The figure shows three views and two pictorial views of one solid part (mm, origin at its lowest corner). Answer the questions. Round coordinates to 2 decimals unless told otherwise and drop trailing zeros. Order: outer loops, then holes, each group sorted by start corner. A loop starts at its lowest first (then second) coordinate and runs counter-clockwise, first axis right, second up. Notation, with made-up numbers: (-27.5, -7.5) - (16.5, -7.5) arc R32 ccw to (16.5, 18.5) - close; hole circle Ø6 at (2.5, 30). An arc over 180 degrees is marked (long way). Answer as a JSON object with one key per item and string values. Group by question number.
Q1. Given pin 1 Ø4 at (x, z) = (152.5, 100) entering from -Y; pin 2 Ø2 at (x, y) = (167, 6) entering from -Z (1 decimal); pin 3 Ø6 at (x, y) = (135.5, 4) entering from +Z; pin 4 Ø2 at (y, z) = (7.5, 119) entering from -X, each flat-ended and moving along its own axis, determine where each tip first touches the part or whether it passes through.
Q2. Consider line 1 (X direction, y = 7.5, z = 170); line 2 (X direction, y = 6.25, z = 100) (1 decimal); line 3 (Z direction, x = 152.5, y = 4.5). Determine where each line is inside the solid, lowest interval first.
Q3. A cutting plane is placed at B-B on z = 188. Determine the outline of the cut face in (x, y).
Q4. A cutting plane is placed at C-C on y = 4.25. Determine the outline of the cut face in (x, z).
Q5. A cutting plane is placed at D-D on z = 231. Determine the outline of the cut face in (x, y).
Q6. A cutting plane is placed at A-A on x = 247.5. Determine the outline of the cut face in (y, z), and give its area (3 significant figures).
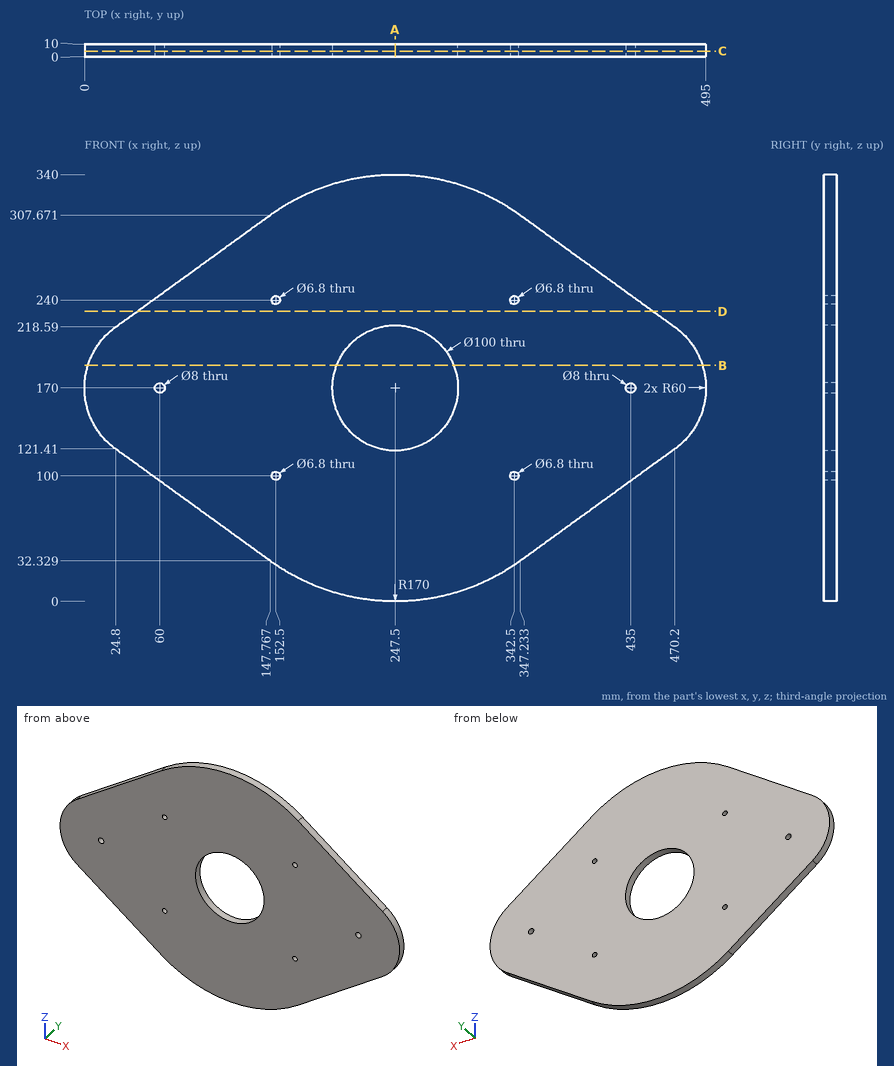
Result set:
{
 "1": {"pin 1": "passes through", "pin 2": "stops at z = 19.7", "pin 3": "stops at z = 300.96", "pin 4": "stops at x = 26.75"},
 "2": {"line 1": "x = 0 to 56, 64 to 197.5, 297.5 to 431, 439 to 495", "line 2": "x = 54.4 to 149.1, 155.9 to 339.1, 345.9 to 440.6", "line 3": "z = 29.02 to 96.6, 103.4 to 236.6, 243.4 to 310.98"},
 "3": {"outline": "(2.76, 0) - (200.85, 0) - (200.85, 10) - (2.76, 10) - close; (294.15, 0) - (492.24, 0) - (492.24, 10) - (294.15, 10) - close"},
 "4": {"outline": "(24.8, 121.41) - (147.77, 32.33) arc R170 ccw to (347.23, 32.33) - (470.2, 121.41) arc R60 ccw to (470.2, 218.59) - (347.23, 307.67) arc R170 ccw to (147.77, 307.67) - (24.8, 218.59) arc R60 ccw to start; hole circle Ø8 at (60, 170); hole circle Ø6.8 at (152.5, 100); hole circle Ø6.8 at (152.5, 240); hole circle Ø100 at (247.5, 170); hole circle Ø6.8 at (342.5, 100); hole circle Ø6.8 at (342.5, 240); hole circle Ø8 at (435, 170)"},
 "5": {"outline": "(41.93, 0) - (453.07, 0) - (453.07, 10) - (41.93, 10) - close"},
 "6": {"outline": "(0, 0) - (10, 0) - (10, 120) - (0, 120) - close; (0, 220) - (10, 220) - (10, 340) - (0, 340) - close", "area": "2,400 mm²"}
}
